Source: CAD feature listing. Evaluate the final solid. Frame: model axes, mm. A direction names the side the tool comes from. Give positions to 0.01 mm unless a question says otherwise; leave off trailing zeros. Answer in a Markdown table with one row per item. Add a question column.
(1) Mould query, pull axis X, two halves, no side actions, for faces 1 (the face through (-69.06, 45.44, 145.58)), 2 (the face through (-3, 25, 210)), 3 (the face through (-225, 25, -3)), 4 (the face through (-65, 41, 50)). Classes: pulls with the +X half, pulls with the -X half, needs draft (parallel to the pull), parting line crosses it, or undercut.
(2) Material intervals for line 1 along Z through (x, y) = (175, 5); line 2 along X through (y, z) = (27.5, 60); line 3 along Z through (x, y) = (147.5, 13.5), sorted ascending.
(3) Set-up query: faces 5 (the face through (3, 0, 3)), 6 (the face through (40.857, 45.437, 48.699)), 7 (the face through (175, 9, -160)). Return all of +Z, -Z, +X, -X, +Y, -Y with unobstructed straight access to the full face (end or side cutting, diameter ignored); none if empty.
(4) Pin query (flat end, axial travel): P1, Ø9.5, axis at x = 175, z = 160, coming from the -Y side; P2, Ø3.5, axis at x = -67, z = 147.5, coming from the +Y side. Return the tip coordinate at first contact, or that it passes through.
Autodesk Inventor part; units mm, degrees
ref_plane "YZ Plane" through (0, 0, 0) normal (1, 0, 0) x (0, 1, 0)
ref_plane "XZ Plane" through (0, 0, 0) normal (0, 1, 0) x (-1, 0, 0)
ref_plane "XY Plane" through (0, 0, 0) normal (0, 0, 1) x (1, 0, 0)
sketch "Sketch1" plane through (0, 0, 0) normal (0, 1, 0) x (-1, 0, 0)
  line L0 (225, 210) -> (-225, 210)
  line L1 (-225, 210) -> (-225, -210)
  line L2 (-225, -210) -> (225, -210)
  line L3 (225, -210) -> (225, 210)
  line L4 (225, -210) -> (-225, 210) construction
  point P0 (0, 0)
  point P1 (0, 0)
  dimension "d0" = 450
  dimension "d1" = 420
extrude "plyta" add sketch "Sketch1" along normal blind 50
sketch "Sketch3" plane through (0, 0, 0) normal (0, -1, 0) x (1, 0, 0)
  line L0 (225, -210) -> (-225, -210)
  line L1 (225, 210) -> (225, -210)
  line L2 (-225, -210) -> (-225, 0)
  line L3 (0, 210) -> (225, 210)
  point P0 (0, 0)
  point P1 (-175, -160)
  point P2 (175, -160)
  point P3 (-175, 160)
  point P4 (175, 160)
  dimension "d18" = 50
  dimension "d19" = 50
  dimension "d20" = 50
  dimension "d21" = 50
hole "Hole2" at (-175, 0, -160) at (175, 0, -160) at (-175, 0, 160) at (175, 0, 160) direction (0, 1, 0) diameter 12 depth 9
sketch "Sketch4" plane through (0, 50, 0) normal (0, 1, 0) x (1, 0, 0)
  line L0 (0, 294) -> (0, -294) construction
  line L1 (-225, -210) -> (225, -210) construction
  point P0 (0, 0)
  point P1 (-65, -150)
  point P2 (35, -150)
  point P3 (-65, -50)
  point P4 (35, -50)
  dimension "d29" = 60
  dimension "d30" = 100
  dimension "d32" = 100
  dimension "d40" = 35
hole "Hole3" at (-65, 50, 150) at (35, 50, 150) at (-65, 50, 50) at (35, 50, 50) direction (0, -1, 0) diameter 12 depth 9
sketch "Sketch5" plane through (0, 50, 0) normal (0, 1, 0) x (1, 0, 0)
  circle A0 centre (197.5, -60) radius 5.75 construction
  circle A1 centre (147.5, -30) radius 5.75 construction
  line L0 (195, 80) -> (215, 80) construction
  line L1 (195, -12.5491) -> (195, 80) construction
  line L2 (150, -12.5491) -> (195, -12.5491) construction
  line L3 (150, 80) -> (150, -12.5491) construction
  line L4 (130, 80) -> (150, 80) construction
  line L5 (130, -80) -> (130, 80) construction
  line L6 (215, -80) -> (130, -80) construction
  line L7 (215, -80) -> (215, 80) construction
  circle A2 centre (147.5, -60) radius 5.75 construction
  circle A3 centre (197.5, -30) radius 5.75 construction
  circle A4 centre (147.5, 150) radius 5.75 construction
  circle A5 centre (197.5, 180) radius 5.75 construction
  line L8 (215, 130) -> (130, 130) construction
  line L9 (215, 130) -> (215, 200) construction
  line L10 (130, 200) -> (215, 200) construction
  line L11 (130, 130) -> (130, 200) construction
  circle A6 centre (147.5, 180) radius 5.75 construction
  circle A7 centre (197.5, 150) radius 5.75 construction
  point P0 (0, 0)
hole "Hole4" at (147.5, 50, 60) at (147.5, 50, 30) at (147.5, 50, -150) at (147.5, 50, -180) at (197.5, 50, -180) at (197.5, 50, -150) at (197.5, 50, 30) at (197.5, 50, 60) direction (0, -1, 0) diameter 8.376 end through all
mirror "Mirror1" about plane through (0, 0, 0) normal (1, 0, 0) of "Hole4"
properties part number "KN-00-01-01" material "Granite, Cut, Polished"
Values follow:
| question | item | result |
|---|---|---|
| 1 | face 1 | undercut |
| 1 | face 2 | needs draft |
| 1 | face 3 | pulls with the -X half |
| 1 | face 4 | undercut |
| 2 | line 1 | z = -210 to -166, -154 to 154, 166 to 210 |
| 2 | line 2 | x = -225 to -201.69, -193.31 to -151.69, -143.31 to 143.31, 151.69 to 193.31, 201.69 to 225 |
| 2 | line 3 | z = -210 to -184.19, -175.81 to -154.19, -145.81 to 25.81, 34.19 to 55.81, 64.19 to 210 |
| 3 | face 5 | +Z, -Z, +X, -X, -Y |
| 3 | face 6 | +Y |
| 3 | face 7 | -Y |
| 4 | P1 | stops at y = 9 |
| 4 | P2 | stops at y = 41 |
